Read the model definition and answer for the solid it produces. Units are mm, in the model's axes. A direction names the side the tool comes from. Coordinates: 2 decimals unless noted, no trailing zeros. Loops run counter-clockwise (first coordinate to the right, second up) from the corner with the lowest first, then second, coordinate; pieces in that order, holes last. Notation, with made-up numbers: M -31,72.5 L -6,72.5 A20 cw -6,76.5 Z; hole C 63,35 d4. An arc over 180 degrees is marked long. Use one line per item in the form item = value. Start each with the question number.
1. The part is cut by section B-B (z = 2.25). Give the vertices of the cut face in (x, y).
2. The part is cut by section D-D (z = 12.25). Give the vertices of the cut face in (x, y), plus the area to 3 significant figures.
3. The part is cut by section A-A (x = 0). Give the vertices of the cut face in (y, z), plus the area to 3 significant figures.
4. The part is cut by section C-C (y = 0). Give the vertices of the cut face in (x, z), plus the area to 3 significant figures.
5. A tool of negligible diameter and unlimited length cuts with its end or side. For faces 4 (the cylindrical face through (0.275, 27.497, 6.902)), 5 (the cylindrical face through (-1.08, 10.12, 12.04)), 6 (the cylindrical face through (6.81, 0.11, 4.95)), from which of +Z, -Z, +X, -X, +Y, -Y can it reach the whole face along a straight path? Write none if from no direction.
6. Find the intervals of material crossed by probe 1 along Y at (x, z) = (0, 13.4); probe 2 along Y at (x, z) = (0, 4); probe 3 along Y at (x, z) = (-1, 2), in increasing order. Write a range as [from, to].
7. For a pull along X with two mould halves and no side action, classify faces 1 (the cylindrical face through (-6.64, 0.11, 4.95)), 2 (the flat face through (1, -18.3, 9)), 3 (the conical face through (0.256, 26.657, 14.84)) as released by +X, released by -X, zero draft, split by the parting line, or undercut.
8. Flat-ended cylindrical pins translate along their axes: pin 1 (1 mm diameter, centred on x = -2, z = 6.5, fed in from -Y); pin 2 (4 mm diameter, centred on x = -3.5, z = 12, fed in from +Y); pin 3 (1.5 mm diameter, centred on y = -20, z = 3, fed in from +X). Find the tip coordinate at first contact, or state that the pin passes through.
from build123d import *

# Parameters (mm, degrees)
SKETCH1_R           = 3.25
BOSS_EXTRUDE1_DEPTH = 15
CUT_EXTRUDE1_REACH  = 27
SKETCH2_R           = 4.95
CHAMFER1_SIZE       = 1
SKETCH3_R           = 5
CUT_EXTRUDE2_DEPTH  = 6
BOSS_EXTRUDE2_DEPTH = 0.95


with BuildPart() as part:
    # Sketch1 → Boss-Extrude1 (new body)
    with BuildSketch(Plane.XY):
        with BuildLine():
            Line((-12.5, 15), (-12.5, -15))
            ThreePointArc((-12.5, -15), (0, -27.5), (12.5, -15))
            Line((12.5, -15), (12.5, 15))
            ThreePointArc((12.5, 15), (0, 27.5), (-12.5, 15))
        make_face()
        with Locations((0, 15)):
            Circle(SKETCH1_R, mode=Mode.SUBTRACT)
        with Locations((0, -15)):
            Circle(SKETCH1_R, mode=Mode.SUBTRACT)
    extrude(amount=BOSS_EXTRUDE1_DEPTH)

    # Sketch2 → Cut-Extrude1 (cut, up to next)
    with BuildSketch(Plane(origin=(12.5, 0, 0), x_dir=(0, 0, -1), z_dir=(1, 0, 0)), mode=Mode.PRIVATE) as cut_extrude1_sk1:
        Circle(SKETCH2_R)
    cut_extrude1_tool1 = extrude(cut_extrude1_sk1.sketch, amount=-CUT_EXTRUDE1_REACH, mode=Mode.PRIVATE) & part.part
    add(cut_extrude1_tool1.solids().sort_by_distance((12.5, 0, 0))[0], mode=Mode.SUBTRACT)

    # Chamfer1
    chamfer1_edges = [part.edges().sort_by_distance(p)[0] for p in [
        (-12.5, 0, 15),
        (0, -27.5, 15),
        (12.5, 0, 15),
        (0, 27.5, 15),
    ]]
    chamfer(chamfer1_edges, length=CHAMFER1_SIZE)

    # Sketch3 → Cut-Extrude2 (cut)
    with BuildSketch(Plane.XY.offset(15)):
        with Locations((0, 15)):
            Circle(SKETCH3_R)
        with Locations((0, -15)):
            Circle(SKETCH3_R)
    extrude(amount=-CUT_EXTRUDE2_DEPTH, mode=Mode.SUBTRACT)

    # Sketch5 → Boss-Extrude2 (add, symmetric)
    with BuildSketch(Plane(origin=(0, 0, 0), x_dir=(0, 0, -1), z_dir=(1, 0, 0))):
        with BuildLine():
            Line((0, 4.5), (0, 4.95))
            ThreePointArc((0, 4.95), (-4.95, 0), (0, -4.95))
            Line((0, -4.95), (0, -4.5))
            ThreePointArc((0, -4.5), (-4.5, 0), (0, 4.5))
        make_face()
    extrude(amount=BOSS_EXTRUDE2_DEPTH, both=True)


solid = part.part
Computed values:
q1.outline = M -12.5,-15 A12.5 ccw 12.5,-15 L 12.5,-4.41 L 0.95,-4.41 L 0.95,-3.9 L -0.95,-3.9 L -0.95,-4.41 L -12.5,-4.41 Z; M -12.5,4.41 L -0.95,4.41 L -0.95,3.9 L 0.95,3.9 L 0.95,4.41 L 12.5,4.41 L 12.5,15 A12.5 ccw -12.5,15 Z; hole C 0,-15 d6.5; hole C 0,15 d6.5
q2.outline = M -12.5,-15 A12.5 ccw 12.5,-15 L 12.5,15 A12.5 ccw -12.5,15 Z; hole C 0,-15 d10; hole C 0,15 d10
q2.area = 1,080 mm²
q3.outline = M -27.5,0 L -18.25,0 L -18.25,9 L -20,9 L -20,15 L -26.5,15 L -27.5,14 Z; M -11.75,0 L -4.5,0 A4.5 cw 4.5,0 L 11.75,0 L 11.75,9 L 10,9 L 10,15 L -10,15 L -10,9 L -11.75,9 Z; M 18.25,0 L 27.5,0 L 27.5,14 L 26.5,15 L 20,15 L 20,9 L 18.25,9 Z
q3.area = 555 mm²
q4.outline = M -12.5,4.95 L -0.95,4.95 L -0.95,4.5 L 0.95,4.5 L 0.95,4.95 L 12.5,4.95 L 12.5,14 L 11.5,15 L -11.5,15 L -12.5,14 Z
q4.area = 251 mm²
q5.face_4 = +Z, -Z, +Y
q5.face_5 = +Z
q5.face_6 = -Z, +X
q6.probe_1 = [-27.5, -20], [-10, 10], [20, 27.5]
q6.probe_2 = [-27.5, -18.25], [-11.75, -2.06], [2.06, 11.75], [18.25, 27.5]
q6.probe_3 = [-27.46, -18.09], [-11.91, -4.53], [4.53, 11.91], [18.09, 27.46]
q7.face_1 = zero draft
q7.face_2 = undercut
q7.face_3 = split by the parting line
q8.pin_1 = -27.41
q8.pin_2 = 27.41
q8.pin_3 = 11.76
